Input: part model. Units: mm. Frame: model coordinates. Coordinates: 2 decimals unless noted, no trailing zeros. Loops run counter-clockwise (first coordinate to the right, second up) from the corner with the lowest first, then second, coordinate; pieces in that order, holes last.
Autodesk Inventor part; units mm, degrees
ref_plane "YZ Plane" through (0, 0, 0) normal (1, 0, 0) x (0, 1, 0)
ref_plane "XZ Plane" through (0, 0, 0) normal (0, 1, 0) x (-1, 0, 0)
ref_plane "XY Plane" through (0, 0, 0) normal (0, 0, 1) x (1, 0, 0)
sketch "Sketch1" plane through (0, 0, 0) normal (1, 0, 0) x (0, 1, 0)
  line L0 (0, 0) -> (50.8, 0)
  line L1 (50.8, 0) -> (50.8, 76.2)
  line L2 (50.8, 76.2) -> (0, 76.2)
  line L3 (0, 76.2) -> (0, 0)
  dimension "d0" = 50.8
  dimension "d1" = 76.2
extrude "Extrusion1" add sketch "Sketch1" along normal blind 3.175
sketch "Sketch2" plane through (3.175, 0, 0) normal (1, 0, 0) x (0, 0, -1)
  line L0 (0, 0) -> (0, 50.8)
  line L1 (0, 50.8) -> (-76.2, 50.8)
  line L2 (-76.2, 50.8) -> (-76.2, 0)
  point P0 (-57.15, 19.05)
  point P1 (-12.7, 38.1)
  dimension "d4" = 12.7
  dimension "d5" = 12.7
  dimension "d6" = 31.75
  dimension "d7" = 19.05
hole "Hole1" at (3.175, 19.05, 57.15) at (3.175, 38.1, 12.7) direction (-1, 0, 0) diameter 3.175 end through all
fillet "Fillet1" radius 6.35 4 edges at (1.5875, 50.8, 76.2) (1.5875, 0, 76.2) (1.5875, 0, 0) (1.5875, 50.8, 0)
properties part number "Base"
Item 1: Section query B-B (z = 12.7). Output: boundary loops of the cut face in (x, y) (1 decimal), then the cut area to 3 significant figures.
Result:
outline: (0, 0) - (3.2, 0) - (3.2, 36.5) - (0, 36.5) - close; (0, 39.7) - (3.2, 39.7) - (3.2, 50.8) - (0, 50.8) - close
area: 151 mm2
Item 2: Contact query for a flat-ended pin moving along its axis: P1, Ø2, axis at y = 27.5, z = 36, coming from the -X side. Output: stop coordinate, or through.
Result:
P1: stops at x = 0
Item 3: Line query: L1, parallel to Z at x = 2.4, y = 38.1; L2, parallel to Z at x = 1.45, y = 19.05; L3, parallel to Y at x = 1.75, z = 57.15. Output: solid intervals per line, ascending.
Result:
L1: z = 0 to 11.11, 14.29 to 76.2
L2: z = 0 to 55.56, 58.74 to 76.2
L3: y = 0 to 17.46, 20.64 to 50.8
Item 4: Section query A-A (y = 19.05). Output: boundary loops of the cut face in (x, z) (1 decimal).
Result:
outline: (0, 0) - (3.2, 0) - (3.2, 55.6) - (0, 55.6) - close; (0, 58.7) - (3.2, 58.7) - (3.2, 76.2) - (0, 76.2) - close
